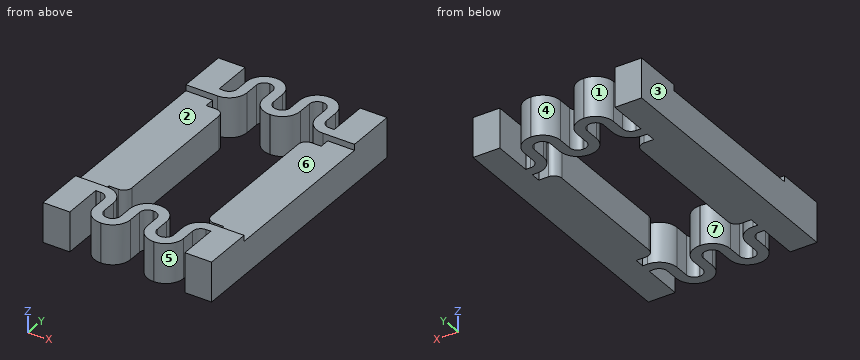
from build123d import *

# Parameters (mm, degrees)
F1_DEPTH = 4
F3_W     = 17
F3_H     = 17
F4_DEPTH = 0.6


with BuildPart() as f1:
    # F0 (on Top) → F1 (new body)
    with BuildSketch(Plane.XY):
        with BuildLine():
            Line((-8.5, 0), (-4, 0))
            Line((-4, 0), (-4, 6.7))
            ThreePointArc((-4, 6.7), (-4.234315, 7.265685), (-4.8, 7.5))
            Line((-4.8, 7.5), (-5.8, 7.5))
            Line((-5.8, 7.5), (-5.8, 8.5))
            Line((-5.8, 8.5), (-5.3, 8.5))
            ThreePointArc((-5.3, 8.5), (-4.027208, 9.027208), (-3.5, 10.3))
            Line((-3.5, 10.3), (-3.5, 11.7))
            ThreePointArc((-3.5, 11.7), (-3.265685, 12.265685), (-2.7, 12.5))
            Line((-2.7, 12.5), (-2.65, 12.5))
            ThreePointArc((-2.65, 12.5), (-2.084315, 12.265685), (-1.85, 11.7))
            Line((-1.85, 11.7), (-1.85, 10.3))
            ThreePointArc((-1.85, 10.3), (-1.322792, 9.027208), (-0.05, 8.5))
            Line((-0.05, 8.5), (0.05, 8.5))
            ThreePointArc((0.05, 8.5), (1.322792, 9.027208), (1.85, 10.3))
            Line((1.85, 10.3), (1.85, 11.7))
            ThreePointArc((1.85, 11.7), (2.084315, 12.265685), (2.65, 12.5))
            Line((2.65, 12.5), (2.7, 12.5))
            ThreePointArc((2.7, 12.5), (3.265685, 12.265685), (3.5, 11.7))
            Line((3.5, 11.7), (3.5, 10.3))
            ThreePointArc((3.5, 10.3), (4.027208, 9.027208), (5.3, 8.5))
            Line((5.3, 8.5), (5.8, 8.5))
            Line((5.8, 8.5), (5.8, 7.5))
            Line((5.8, 7.5), (4.8, 7.5))
            ThreePointArc((4.8, 7.5), (4.234315, 7.265685), (4, 6.7))
            Line((4, 6.7), (4, 0))
            Line((4, 0), (8.5, 0))
            Line((8.5, 0), (8.5, 13.5))
            Line((8.5, 13.5), (5.8, 13.5))
            Line((5.8, 13.5), (5.8, 9.5))
            Line((5.8, 9.5), (5.3, 9.5))
            ThreePointArc((5.3, 9.5), (4.734315, 9.734315), (4.5, 10.3))
            Line((4.5, 10.3), (4.5, 11.7))
            ThreePointArc((4.5, 11.7), (3.972792, 12.972792), (2.7, 13.5))
            Line((2.7, 13.5), (2.65, 13.5))
            ThreePointArc((2.65, 13.5), (1.377208, 12.972792), (0.85, 11.7))
            Line((0.85, 11.7), (0.85, 10.3))
            ThreePointArc((0.85, 10.3), (0.615685, 9.734315), (0.05, 9.5))
            Line((0.05, 9.5), (-0.05, 9.5))
            ThreePointArc((-0.05, 9.5), (-0.615685, 9.734315), (-0.85, 10.3))
            Line((-0.85, 10.3), (-0.85, 11.7))
            ThreePointArc((-0.85, 11.7), (-1.377208, 12.972792), (-2.65, 13.5))
            Line((-2.65, 13.5), (-2.7, 13.5))
            ThreePointArc((-2.7, 13.5), (-3.972792, 12.972792), (-4.5, 11.7))
            Line((-4.5, 11.7), (-4.5, 10.3))
            ThreePointArc((-4.5, 10.3), (-4.734315, 9.734315), (-5.3, 9.5))
            Line((-5.3, 9.5), (-5.8, 9.5))
            Line((-5.8, 9.5), (-5.8, 13.5))
            Line((-5.8, 13.5), (-8.5, 13.5))
            Line((-8.5, 13.5), (-8.5, 0))
        make_face()
    extrude(amount=F1_DEPTH)

    # F2: F1 across plane


with BuildPart() as f1_1:
    add(f1.part)
    add(f1.part.mirror(Plane.XZ))

    # F3 (on face) → F4 (cut)
    with BuildSketch(Plane.XY.offset(4)):
        Rectangle(F3_W, F3_H)
    extrude(amount=-F4_DEPTH, mode=Mode.SUBTRACT)


solid = f1_1.part
Geometry: final body of the model. Coordinates: model frame, mm. Face numbers are marked on the shaded views. A direction names the side the tool comes from. Give positions to 0.01 mm unless a question says otherwise; leave off trailing zeros. Write each loop counter-clockwise with the first axis right and the second up, starting at its lowest first coordinate (ties: lowest second). Pieces come first, ordered by that corner, then holes.
(1) Cut plane C-C, the plane x = -0.5. Return loops of the section in (y, z).
(2) Mould query, pull axis X, two halves, no side actions, for the marked faces 1, 2 and 3. Classes: released by +X, released by -X, zero draft, split by the parting line, or undercut.
(3) Cut plane B-B, the plane y = 11. Return loops of the section in (x, z).
(4) Cut plane A-A, the plane y = 2.5. Return loops of the section in (x, z), then the cut area to 3 significant figures.
(5) Ray query, line 1 (Y direction, x = -2.75, z = 1); line 2 (X direction, y = -11.5, z = 2.5); line 3 (X direction, y = -0.75, z = 2.6). Return the intervals inside material, ascending.
(6) Cut plane D-D, the plane y = -10. Return loops of the section in (x, z).
(7) Access query for the marked faces 4, 5, 6 and 7. Directions: +Z, -Z, +X, -X, +Y, -Y. A direction counts if a zero-diameter tool reaches every point of the face in a straight line with its end or side. Return the directions, or none.
(8) First-contact query: P1, Ø1.3, axis at x = 7, y = 1, coming from the +Z side; P2, Ø1.5, axis at x = 1.5, z = 1, coming from the +Y side (3 decimals); P3, Ø0.5, axis at x = 5.5, z = 2.5, coming from the +Y side. Flat tips, straight axial feed; report the tip coordinate or a pass-through.
Values follow:
1. outline: (-9.64, 0) - (-8.56, 0) - (-8.56, 4) - (-9.64, 4) - close; (8.56, 0) - (9.64, 0) - (9.64, 4) - (8.56, 4) - close
2. face 1: undercut
2. face 2: zero draft
2. face 3: released by -X
3. outline: (-8.5, 0) - (-5.8, 0) - (-5.8, 4) - (-8.5, 4) - close; (-4.5, 0) - (-3.5, 0) - (-3.5, 4) - (-4.5, 4) - close; (-1.85, 0) - (-0.85, 0) - (-0.85, 4) - (-1.85, 4) - close; (0.85, 0) - (1.85, 0) - (1.85, 4) - (0.85, 4) - close; (3.5, 0) - (4.5, 0) - (4.5, 4) - (3.5, 4) - close; (5.8, 0) - (8.5, 0) - (8.5, 4) - (5.8, 4) - close
4. outline: (-8.5, 0) - (-4, 0) - (-4, 3.4) - (-8.5, 3.4) - close; (4, 0) - (8.5, 0) - (8.5, 3.4) - (4, 3.4) - close
4. area: 30.6 mm2
5. line 1: y = -13.5 to -12.5, 12.5 to 13.5
5. line 2: x = -8.5 to -5.8, -4.5 to -3.5, -1.85 to -0.85, 0.85 to 1.85, 3.5 to 4.5, 5.8 to 8.5
5. line 3: x = -8.5 to -4, 4 to 8.5
6. outline: (-8.5, 0) - (-5.8, 0) - (-5.8, 4) - (-8.5, 4) - close; (-4.56, 0) - (-3.53, 0) - (-3.53, 4) - (-4.56, 4) - close; (-1.82, 0) - (-0.79, 0) - (-0.79, 4) - (-1.82, 4) - close; (0.79, 0) - (1.82, 0) - (1.82, 4) - (0.79, 4) - close; (3.53, 0) - (4.56, 0) - (4.56, 4) - (3.53, 4) - close; (5.8, 0) - (8.5, 0) - (8.5, 4) - (5.8, 4) - close
7. face 4: +Z, -Z, +Y
7. face 5: +Z, -Z, -Y
7. face 6: +Z, +X, -X
7. face 7: +Z, -Z
8. P1: stops at z = 3.4
8. P2: stops at y = 13.455
8. P3: stops at y = 9.5
